Part print with two shaded views. Sizes in mm from the minimum x, y, z corner. A direction names the side the tool comes from. Give positions to 0.01 mm unless a question says otherwise; leave off trailing zeros. Write each loop counter-clockwise with the first axis right and the second up, starting at its lowest first coordinate (ties: lowest second). Pieces come first, ordered by that corner, then holes. Notation, with made-up numbers: (-17, 1) - (-1, 1) arc R12 ccw to (-1, 14) - close; hole circle Ø4 at (85.25, 63). An arc over 180 degrees is marked (long way). Answer as a JSON object with one key per item and string values.
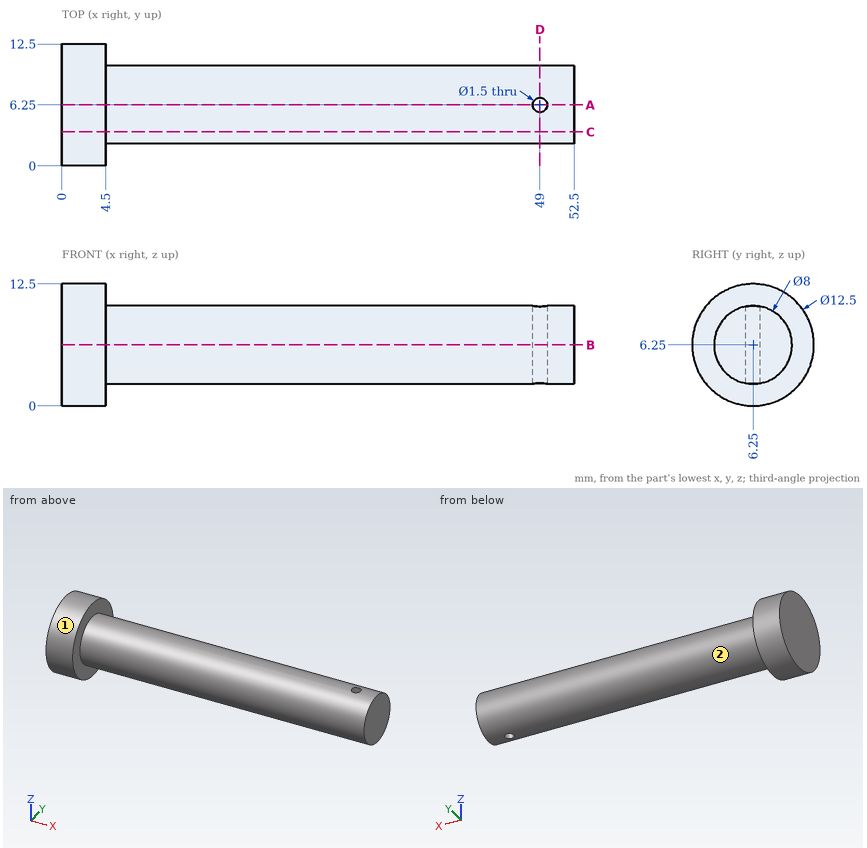
(1) Saw through at D-D, the plane x = 49. Give the cut face in (y, z).
Answer key:
{"outline": "(5.5, 2.32) - (5.5, 10.18) arc R4 ccw to start; (7, 2.32) arc R4 ccw to (7, 10.18) - close"}
(2) Saw through at C-C, the plane y = 3.5. Give the cut face in (x, z), and give its area (3 significant figures).
Answer key:
{"outline": "(0, 0.64) - (4.5, 0.64) - (4.5, 3.35) - (52.5, 3.35) - (52.5, 9.15) - (4.5, 9.15) - (4.5, 11.86) - (0, 11.86) - close", "area": "329 mm²"}
(3) Flat gauge pins, fed straight in: P1, Ø5, axis at x = 33.5, y = 7, coming from the +Z side; P2, Ø3, axis at x = 34.5, z = 8, coming from the +Y side; P3, Ø5, axis at x = 41.5, y = 3, coming from the -Z side. Where does each tip first touch, or does it go through?
Answer key:
{"P1": "stops at z = 10.25", "P2": "stops at y = 10.24", "P3": "stops at z = 2.32"}
(4) 3-axis set-ups, long thin cutter, end or side, ignore diameter. For the marked faces 1 and 2: which of +Z, -Z, +X, -X, +Y, -Y reach the whole face in a straight line?
Answer key:
{"face 1": "+X, -X", "face 2": "+X"}
(5) Probe L1, parallel to X at y = 6.25, z = 7.5; L2, parallel to X at y = 4, z = 10.75; L3, parallel to Y at x = 49, z = 4.5. List the from-to ranges inside material, lowest first. Write a range as [from, to].
Answer key:
{"L1": "x = [0, 48.25], [49.75, 52.5]", "L2": "x = [0, 4.5]", "L3": "y = [2.65, 5.5], [7, 9.85]"}
(6) Saw through at A-A, the plane y = 6.25. Give the cut face in (x, z).
Answer key:
{"outline": "(0, 0) - (4.5, 0) - (4.5, 2.25) - (48.25, 2.25) - (48.25, 10.25) - (4.5, 10.25) - (4.5, 12.5) - (0, 12.5) - close; (49.75, 2.25) - (52.5, 2.25) - (52.5, 10.25) - (49.75, 10.25) - close"}
(7) Saw through at B-B, the plane z = 6.25. Give the cut face in (x, y), and give its area (3 significant figures).
Answer key:
{"outline": "(0, 0) - (4.5, 0) - (4.5, 2.25) - (52.5, 2.25) - (52.5, 10.25) - (4.5, 10.25) - (4.5, 12.5) - (0, 12.5) - close; hole circle Ø1.5 at (49, 6.25)", "area": "438 mm²"}
